For this review, take the finished solid that the model builds, in its own axes (mm). Face numbers are marked on the shaded views. A direction names the side the tool comes from. Give positions to 0.01 mm unless a question says otherwise; leave off trailing zeros. Order: outer loops, then holes, each group sorted by start corner. A loop starts at its lowest first (then second) coordinate and runs counter-clockwise, first axis right, second up.
from build123d import *

# Parameters (mm, degrees)
F0_W      = 56
F0_H      = 48
F1_DEPTH  = 31
F2_R      = 0.475
F2_R_2    = 0.425
F3_DEPTH  = 2
F6_DEPTH  = 15.95
F7_DEPTH  = 15.95
F8_R      = 2.5
F9_DEPTH  = 10
F11_DEPTH = 56.001
F12_R     = 2
F13_DEPTH = 20
F14_R     = 4
F15_DEPTH = 14


with BuildPart() as f1:
    # F0 (on Top) → F1 (new body)
    with BuildSketch(Plane.XY):
        with Locations((28, 24)):
            Rectangle(F0_W, F0_H)
    extrude(amount=-F1_DEPTH)

    # F2 (on Top) → F3 (join)
    with BuildSketch(Plane.XY):
        with Locations((18.3, 24)):
            Circle(F2_R)
        with Locations((37.7, 24)):
            Circle(F2_R_2)
    extrude(amount=F3_DEPTH)

    # F4 (on face) → F6 (cut)
    with BuildSketch(Plane.YZ.offset(56)):
        Polygon((25, 0), (23, 0), (23, -4), (21, -4), (21, -6), (27, -6), (27, -4), (25, -4), align=None)
    extrude(amount=-F6_DEPTH, mode=Mode.SUBTRACT)

    # F5 (on face) → F7 (cut)
    with BuildSketch(Plane(origin=(0, 0, 0), x_dir=(0, -1, 0), z_dir=(-1, 0, 0))):
        Polygon((-23, 0), (-25, 0), (-25, -4), (-27, -4), (-27, -6), (-21, -6), (-21, -4), (-23, -4), align=None)
    extrude(amount=-F7_DEPTH, mode=Mode.SUBTRACT)

    # F8 (on face) → F9 (cut)
    with BuildSketch(Plane.XZ):
        with Locations((18, -5)):
            Circle(F8_R)
    extrude(amount=-F9_DEPTH, mode=Mode.SUBTRACT)

    # F10 (on face) → F11 (cut, through all)
    with BuildSketch(Plane.YZ.offset(56)):
        Polygon((5, 0), (0, 0), (-4.974183, 0), (-4.974183, -37.207626), (53.682573, -37.207626), (53.682573, 0), (48, 0), (43, 0), (43, -21), (48, -21), (48, -31), (38, -31), (38, -29), (10, -29), (10, -31), (0, -31), (0, -21), (5, -21), align=None)
    extrude(amount=-F11_DEPTH, mode=Mode.SUBTRACT)

    # F12 (on face) → F13 (cut)
    with BuildSketch(Plane(origin=(0, 43, 0), x_dir=(-1, 0, 0), z_dir=(0, 1, 0))):
        with Locations((-48.05, -5)):
            Circle(F12_R)
        with Locations((-7.95, -5)):
            Circle(F12_R)
    extrude(amount=-F13_DEPTH, mode=Mode.SUBTRACT)

    # F14 (on face) → F15 (cut)
    with BuildSketch(Plane(origin=(0, 43, 0), x_dir=(-1, 0, 0), z_dir=(0, 1, 0))):
        with Locations((-48.05, -5)):
            Circle(F14_R)
        with Locations((-7.95, -5)):
            Circle(F14_R)
    extrude(amount=-F15_DEPTH, mode=Mode.SUBTRACT)


solid = f1.part
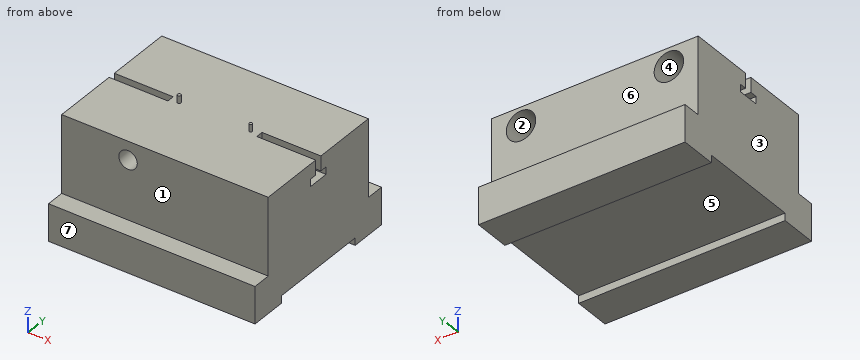
1) We need section A-A on x = 7.95. Give the boundary of the cut face in (y, z).
Answer sheet:
outline: (0, -31) - (10, -31) - (10, -29) - (38, -29) - (38, -31) - (48, -31) - (48, -21) - (43, -21) - (43, -9) - (29, -9) - (29, -7) - (23, -7) - (23, -6) - (21, -6) - (21, -4) - (23, -4) - (23, 0) - (5, 0) - (5, -21) - (0, -21) - close; (25, -3) - (29, -3) - (29, -1) - (43, -1) - (43, 0) - (25, 0) - close
2) Draft analysis for pull direction X (two halves, no side actions). For the marked faces 1, 2, 3 and 4, state which applies: +X half, -X half, draft (parallel to the pull), parting line (faces both ways), or undercut.
Answer sheet:
face 1: draft
face 2: undercut
face 3: -X half
face 4: undercut
3) To check wall thickness, follow line 1 (Z direction, x = 18, y = 6); line 2 (Z direction, x = 48, y = 26); line 3 (Y direction, x = 6, z = -10.5). State the ranges of each line that lie inside material, in increasing order.
Answer sheet:
line 1: z = -31 to -7.5, -2.5 to 0
line 2: z = -29 to -7, -3 to 0
line 3: y = 5 to 43
4) Clearance check with flat-ended pins moving along their axes: pin 1 (1.6 mm diameter, centred on x = 36, z = -30.5, fed in from -Y); pin 2 (3 mm diameter, centred on x = 46.5, y = 25.5, fed in from +Z); pin 3 (1 mm diameter, centred on x = 10.5, z = -5, fed in from +Y); pin 4 (5.5 mm diameter, centred on x = 18.5, y = 46, fed in from +Z). State where each tip first meets the part, or that it passes through.
Answer sheet:
pin 1: stops at y = 0
pin 2: stops at z = 0
pin 3: stops at y = 29
pin 4: stops at z = -21
5) Tool access review of the marked faces 5, 6 and 7: name each direction out of +Z, -Z, +X, -X, +Y, -Y from which nothing blocks a thin tool from reaching the whole face with its end or side.
Answer sheet:
face 5: -Z, +X, -X
face 6: +Z, +X, -X, +Y
face 7: +Z, -Z, +X, -X, -Y
6) We need section D-D on y = 40.5. Give the boundary of the cut face in (x, z), then the cut area to 3 significant figures.
Answer sheet:
outline: (0, -31) - (56, -31) - (56, 0) - (0, 0) - close; hole circle Ø8 at (7.95, -5); hole circle Ø8 at (48.05, -5)
area: 1,640 mm2
7) We need section B-B on y = 8. Give the boundary of the cut face in (x, z), then the cut area to 3 significant figures.
Answer sheet:
outline: (0, -31) - (56, -31) - (56, 0) - (0, 0) - close; hole circle Ø5 at (18, -5)
area: 1,720 mm2
8) We need section C-C on z = -5. Count the separate pieces of the cut face and the enclosed holes in it, then the cut area to 3 significant figures.
Answer sheet:
separate pieces: 3
enclosed holes: 0
area: 1,670 mm2
